Geometry: final body of the model. Coordinates: model frame, mm. A direction names the side the tool comes from. Round coordinates to 2 decimals unless told otherwise and drop trailing zeros. Write each loop counter-clockwise with the first axis right and the second up, starting at its lowest first coordinate (ties: lowest second). Pieces come first, ordered by that corner, then holes. Notation, with made-up numbers: M 8.25,4 L 51.25,4 A20 ccw 51.25,16 Z; hole C 44.5,14 d5. An arc over 180 degrees is marked long. Use one line per item in the form item = value. Start each with the question number.
Item 1: Ray query, probe 1 along Z at (x, y) = (0.5, -0.5); probe 2 along Y at (x, z) = (1.25, 12.5); probe 3 along Y at (x, z) = (2.75, 9). Return the intervals inside material, ascending.
Item 2: Reachability of faces 1 (the flat face through (0, 0, 16.272)), 2 (the cylindrical face through (2.933, 0.81, 7.821)) from +Z, -Z, +X, -X, +Y, -Y: full face, straight path, thin tool, end or side. Return the list, or none.
Item 3: Section query B-B (x = 0). Return loops of the section in (y, z).
Item 4: Pull-direction query (Z, two-part tool) for faces 3 (the cylindrical face through (-0.044, -0.832, 11.276)), 4 (the cylindrical face through (-0.86, -3.86, -7.83)), 5 (the flat face through (0, 0, -16.272)), 6 (the flat face through (-1, 3, -0.397)); classes: pulls with the +Z half, pulls with the -Z half, needs draft (parallel to the pull), parting line crosses it, or undercut.
Item 5: Section query D-D (z = 4.5). Return loops of the section in (x, y) (3 decimals).
Item 6: Section query C-C (z = -1.5). Return loops of the section in (x, y), and give its area (3 significant figures).
Item 7: Section query A-A (y = 0). Return loops of the section in (x, z), and give its area (3 significant figures).
Item 8: Pin query (flat end, axial travel): pin 1 Ø1 at (x, z) = (1.5, 0) entering from +Y; pin 2 Ø3.5 at (y, z) = (-0.41, 12.3) entering from -X (3 decimals). Return the tip coordinate at first contact, or that it passes through.
from build123d import *

# Parameters (mm, degrees)
SKETCH1_R                   = 3.95605
BASE_EXTRUDE_DEPTH          = 16.271875
CHAMFER1_SIZE               = 0.79375
SILHOUETTE_W                = 16.66875
SILHOUETTE_H                = 1.18745
LOCKING_PIN_HOLE_DEPTH      = 18.206817812
LOCKING_PIN_HOLE_DEPTH_BACK = 18.206817812
SKETCH5_R                   = 1.112153358


with BuildPart() as part:
    # Sketch1 → Base-Extrude (new, symmetric)
    with BuildSketch(Plane.XY):
        Circle(SKETCH1_R)
    extrude(amount=BASE_EXTRUDE_DEPTH, both=True)

    # Chamfer1
    chamfer1_edges = [part.edges().sort_by_distance(p)[0] for p in [
        (-3.95605, 0, -16.271875),
    ]]
    chamfer(chamfer1_edges, length=CHAMFER1_SIZE)

    # Silhouette → Cut-Revolve1 (revolve, cut)
    with BuildSketch(Plane(origin=(0, 0, 0), x_dir=(0, 0, -1), z_dir=(1, 0, 0)), mode=Mode.PRIVATE) as cut_revolve1_sk:
        with Locations((-7.9375, 3.362325)):
            Rectangle(SILHOUETTE_W, SILHOUETTE_H)
    revolve(cut_revolve1_sk.sketch.rotate(Axis((0, -0.4064, 13.51559633), (0, 0, -1)), 90), axis=Axis((0, -0.4064, 13.51559633), (0, 0, -1)), mode=Mode.SUBTRACT)

    # Sketch5 → Locking pin hole (cut, two sides: drawn at the far end of the back side and taken through both)
    with BuildSketch(Plane(origin=(0, 0, 0), x_dir=(0, 0, -1), z_dir=(1, 0, 0)).offset(-LOCKING_PIN_HOLE_DEPTH_BACK)):
        with Locations((-12.303125, -0.4064)):
            Circle(SKETCH5_R)
    extrude(amount=LOCKING_PIN_HOLE_DEPTH + LOCKING_PIN_HOLE_DEPTH_BACK, mode=Mode.SUBTRACT)


solid = part.part
Working result:
q1.probe_1 = -16.27 to 11.19, 13.41 to 16.27
q1.probe_2 = -3.32 to -1.5, 0.69 to 2.51
q1.probe_3 = -1.99 to 1.18
q2.face_1 = +Z, +X, -X, +Y, -Y
q2.face_2 = +Z
q3.outline = M -3.96,-15.48 L -3.16,-16.27 L 3.16,-16.27 L 3.96,-15.48 L 3.96,-0.4 L 2.77,-0.4 L 2.77,16.27 L -3.58,16.27 L -3.58,-0.4 L -3.96,-0.4 Z; hole C -0.41,12.3 d2.22
q4.face_3 = undercut
q4.face_4 = needs draft
q4.face_5 = pulls with the -Z half
q4.face_6 = pulls with the +Z half
q5.outline = C 0,-0.406 d6.35
q6.outline = C 0,0 d7.91
q6.area = 49.2 mm²
q7.outline = M -3.96,-15.48 L -3.16,-16.27 L 3.16,-16.27 L 3.96,-15.48 L 3.96,-0.4 L 3.15,-0.4 L 3.15,11.27 L -3.15,11.27 L -3.15,-0.4 L -3.96,-0.4 Z; M -3.15,13.34 L 3.15,13.34 L 3.15,16.27 L -3.15,16.27 Z
q7.area = 217 mm²
q8.pin_1 = 3.77
q8.pin_2 = -3.175
